```python
from build123d import *

# Parameters (mm, degrees)
F6_W     = 76.2
F6_H     = 76.2
F0_DEPTH = 76.2
F1_D     = 25.4
F8_D     = 25.4
F4_D     = 25.4


with BuildPart() as f0:
    # F6 (on Right) → F0 (new body)
    with BuildSketch(Plane.YZ):
        Rectangle(F6_W, F6_H)
    extrude(amount=-F0_DEPTH)

    # F1 (through all)
    with Locations(Plane.XZ.offset(38.1)):
        with Locations((-38.1, 0)):
            Hole(F1_D / 2)

    # F8 (through all)
    with Locations(Plane.XY.offset(38.1)):
        with Locations((-38.1, 0)):
            Hole(F8_D / 2)

    # F4 (through all)
    with Locations(Plane.YZ):
        with Locations((0, 0)):
            Hole(F4_D / 2)


solid = f0.part
```
The listing builds one solid part. Answer for the finished solid, in the listing's coordinates (mm). Coordinates: 2 decimals unless noted, no trailing zeros. Write each loop counter-clockwise with the first axis right and the second up, starting at its lowest first coordinate (ties: lowest second). Pieces come first, ordered by that corner, then holes. Notation, with made-up numbers: (5, 15.25) - (53, 15.25) arc R22 ccw to (53, 41.25) - close; hole circle Ø2 at (0, 26). An arc over 180 degrees is marked (long way). One line per item, written item: value.
1) For a pull along Y with two mould halves and no side action, classify faces 1 (the flat face through (-38, -17, -38.1)), 2 (the flat face through (-38, 38.1, -17)), 3 (the cylindrical face through (-25.412, 0.558, 23.336)), 4 (the cylindrical face through (-28.74, 8.583, -23.744)) as pulls with the +Y half, pulls with the -Y half, needs draft (parallel to the pull), parting line crosses it, or undercut.
Geometry check:
face 1: needs draft
face 2: pulls with the +Y half
face 3: undercut
face 4: undercut
2) Find section B-B (y = 0). Give the vertices of the cut face in (x, z), and give its area (3 significant figures).
Geometry check:
outline: (-76.2, -38.1) - (-50.8, -38.1) - (-50.8, -12.7) - (-76.2, -12.7) - close; (-76.2, 12.7) - (-50.8, 12.7) - (-50.8, 38.1) - (-76.2, 38.1) - close; (-25.4, -38.1) - (0, -38.1) - (0, -12.7) - (-25.4, -12.7) - close; (-25.4, 12.7) - (0, 12.7) - (0, 38.1) - (-25.4, 38.1) - close
area: 2,580 mm2
3) Find section A-A (x = -38.1). Give the vertices of the cut face in (y, z), and give its area (3 significant figures).
Geometry check:
outline: (-38.1, -38.1) - (-12.7, -38.1) - (-12.7, -12.7) - (-38.1, -12.7) - close; (-38.1, 12.7) - (-12.7, 12.7) - (-12.7, 38.1) - (-38.1, 38.1) - close; (12.7, -38.1) - (38.1, -38.1) - (38.1, -12.7) - (12.7, -12.7) - close; (12.7, 12.7) - (38.1, 12.7) - (38.1, 38.1) - (12.7, 38.1) - close
area: 2,580 mm2
4) Find section C-C (z = 21.5). Give the vertices of the cut face in (x, y), and give its area (3 significant figures).
Geometry check:
outline: (-76.2, -38.1) - (0, -38.1) - (0, 38.1) - (-76.2, 38.1) - close; hole circle Ø25.4 at (-38.1, 0)
area: 5,300 mm2
5) Find section D-D (x = -23). Give the vertices of the cut face in (y, z).
Geometry check:
outline: (-38.1, -38.1) - (38.1, -38.1) - (38.1, 38.1) - (-38.1, 38.1) - close; hole circle Ø25.4 at (0, 0)
6) Consider line 1 along X through (y, z) = (-21.25, 0); line 2 along Y through (x, z) = (-38.1, 27); line 3 along X through (y, z) = (-25, -9). Determine where each line is inside the solid, lowest interval first. Write a range as from..to.
Geometry check:
line 1: x = -76.2..-50.8, -25.4..0
line 2: y = -38.1..-12.7, 12.7..38.1
line 3: x = -76.2..-47.06, -29.14..0
7) This flat-tipped pin is pushed along its axis until it touches: pin 1 Ø23 at (x, y) = (-38.1, 0) entering from +Z. Where does it stop, or does it pass through?
Geometry check:
pin 1: passes through
